Source: CAD feature listing. Evaluate the final solid. Frame: model axes, mm. Face numbers are marked on the shaded views. Round coordinates to 2 decimals unless told otherwise and drop trailing zeros. Write each loop counter-clockwise with the first axis right and the second up, starting at its lowest first coordinate (ties: lowest second). Pieces come first, ordered by that corner, then holes. Notation, with made-up numbers: M -17,28.25 L 10,28.25 A30 cw 10,67.25 Z; hole C 4.5,27 d7. An arc over 180 degrees is marked long. Use a Markdown table: item, result.
```python
from build123d import *

# Parameters (mm, degrees)
BOSS_EXTRU_1_DEPTH      = 10
ESQUISSE2_R             = 1.55
ENL_V_MAT_EXTRU_1_DEPTH = 7


with BuildPart() as part:
    # Esquisse1 → Boss.-Extru.1 (new body)
    with BuildSketch(Plane(origin=(0, 0, 0), x_dir=(1, 0, 0), z_dir=(0, 1, 0))):
        Polygon((-28.5, -5), (28.5, -5), (28.5, 7), (19, 7), (19, 5), (-19, 5), (-19, 7), (-28.5, 7), align=None)
    extrude(amount=BOSS_EXTRU_1_DEPTH)

    # Esquisse2 → Enlèv. mat.-Extru.1 (cut)
    with BuildSketch(Plane(origin=(0, 0, -7), x_dir=(-1, 0, 0), z_dir=(0, 0, -1))):
        with Locations((-23.5, 5)):
            Circle(ESQUISSE2_R)
    enl_v_mat_extru_1 = extrude(amount=-ENL_V_MAT_EXTRU_1_DEPTH, mode=Mode.SUBTRACT)

    # Esquisse4 → Fraisage pour vis à tête fraisée à 6 pans creux M31 (revolve, cut)
    with BuildSketch(Plane(origin=(14.5, 5, 5), x_dir=(0, -1, 0), z_dir=(1, 0, 0))):
        Polygon((0, 0), (0, 12), (1.6, 12), (1.6, 1.7), (2.9, 0.4), (2.9, 0), align=None)
    fraisage_pour_vis_t_te_frais_e_6_pan = revolve(axis=Axis((14.5, 5, 11.35), (0, 0, -1)), mode=Mode.SUBTRACT)

    # Symétrie1: Enlèv. mat.-Extru.1, Fraisage pour vis à tête fraisée à 6 pans creux M31 across plane
    add(enl_v_mat_extru_1.mirror(Plane(origin=(0, 0, 0), x_dir=(0, 0, 1), z_dir=(1, 0, 0))), mode=Mode.SUBTRACT)
    add(fraisage_pour_vis_t_te_frais_e_6_pan.mirror(Plane(origin=(0, 0, 0), x_dir=(0, 0, 1), z_dir=(1, 0, 0))), mode=Mode.SUBTRACT)


solid = part.part
```
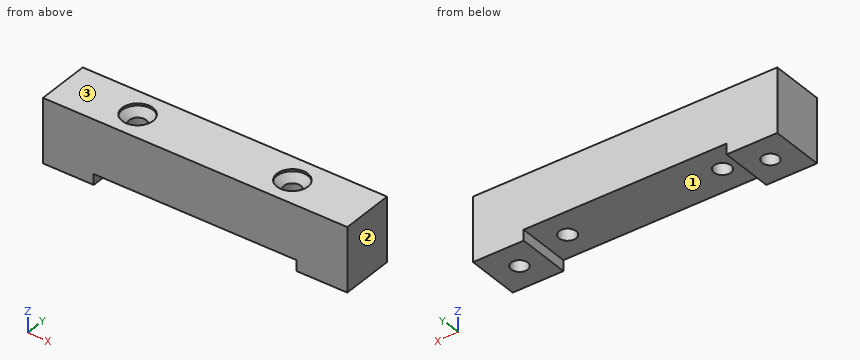
Q1. First-contact query: pin 1 Ø4.5 at (x, y) = (14.5, 5) entering from -Z; pin 2 Ø1.5 at (x, y) = (24, 5) entering from -Z; pin 3 Ø4 at (x, y) = (-14.5, 5) entering from +Z. Flat tips, straight axial feed; report the tip coordinate or a pass-through.
Results are:
| item | result |
|---|---|
| pin 1 | z = -5 |
| pin 2 | z = 0 |
| pin 3 | z = 3.7 |
Q2. Line query: L1, parallel to X at y = 5, z = 0.5; L2, parallel to X at y = 7.5, z = -6.5; L3, parallel to Y at x = 14.5, z = 4.8. Output: solid intervals per line, ascending.
Results are:
| item | result |
|---|---|
| L1 | -28.5 to -16.1, -12.9 to 12.9, 16.1 to 28.5 |
| L2 | -28.5 to -19, 19 to 28.5 |
| L3 | 0 to 2.1, 7.9 to 10 |
Q3. Section C-C on z = -1.5. Return loops of the section in (x, y), plus the area to 3 significant figures.
Results are:
| item | result |
|---|---|
| outline | M -28.5,0 L 28.5,0 L 28.5,10 L -28.5,10 Z; hole C -23.5,5 d3.1; hole C -14.5,5 d3.2; hole C 14.5,5 d3.2; hole C 23.5,5 d3.1 |
| area | 539 mm^2 |
Q4. Mould query, pull axis X, two halves, no side actions, for the marked faces 1, 2 and 3. Classes: +X half, -X half, draft (parallel to the pull), parting line (faces both ways), or undercut.
Results are:
| item | result |
|---|---|
| face 1 | undercut |
| face 2 | +X half |
| face 3 | draft |
Q5. Section D-D on x = 23.5. Return loops of the section in (y, z).
Results are:
| item | result |
|---|---|
| outline | M 0,-7 L 3.45,-7 L 3.45,0 L 6.55,0 L 6.55,-7 L 10,-7 L 10,5 L 0,5 Z |
Q6. Section A-A on z = -5.5. Return loops of the section in (x, y), plus the area to 3 significant figures.
Results are:
| item | result |
|---|---|
| outline | M -28.5,0 L -19,0 L -19,10 L -28.5,10 Z; M 19,0 L 28.5,0 L 28.5,10 L 19,10 Z; hole C -23.5,5 d3.1; hole C 23.5,5 d3.1 |
| area | 175 mm^2 |
Q7. Section B-B on x = -14.5. Return loops of the section in (y, z), plus the area to 3 significant figures.
Results are:
| item | result |
|---|---|
| outline | M 0,-5 L 3.4,-5 L 3.4,3.3 L 2.1,4.6 L 2.1,5 L 0,5 Z; M 6.6,-5 L 10,-5 L 10,5 L 7.9,5 L 7.9,4.6 L 6.6,3.3 Z |
| area | 65.3 mm^2 |
